For this review, take the finished solid that the model builds, in its own axes (mm). A direction names the side the tool comes from. Coordinates: 2 decimals unless noted, no trailing zeros. Order: outer loops, then holes, each group sorted by start corner. A loop starts at its lowest first (then second) coordinate and runs counter-clockwise, first axis right, second up. Notation, with made-up numbers: (78, 26) - (133, 26) arc R37 cw to (133, 62) - close; hole circle Ø6 at (40, 33). An arc over 180 degrees is marked (long way). One line per item, written item: value. Start each with the question number.
(1) Consider section B-B on z = 50.5. Write out the cut boundary in (x, y), then the cut area to 3 significant figures.
(2) To check wall thickness, follow line 1 along X through (y, z) = (9.5, 38); line 2 along Z through (x, y) = (-91.5, 3.5); line 3 along X through (y, z) = (30.5, 66.5). State the ranges of each line that lie inside material, in increasing order.
(3) For faces 4 (the flat face through (-119, 37, 75)), 5 (the flat face through (-120, 31, 16.891)), 6 (the flat face through (-95, 23.75, 66)), 7 (the flat face through (-92.412, 11.4, 31.9)), 8 (the flat face through (-138.162, 20, 46)), list the 3-axis set-ups (+Z, -Z, +X, -X, +Y, -Y) from which the entire face can be reached by the end or side of a thin tool; tool diameter is ignored.
(4) Consider section D-D on z = 19.5. Count the separate pieces of the cut face and the enclosed holes in it, then the cut area to 3 significant figures.
(5) Mouldability with a two-part tool opening along X and no side actions: class faces 1 (the flat face through (-136.412, 5, 10)), 2 (the flat face through (-113, 11, 74.391)), 3 (the flat face through (-93, 32, 16.641)) as released by +X, released by -X, zero draft, split by the parting line, or undercut.
(6) Consider section C-C on x = -152. Write out the cut boundary in (y, z), then the cut area to 3 significant figures.
(7) Consider section A-A on y = 34. Write out the cut boundary in (x, z), then the cut area to 3 significant figures.
(8) Clearance check with flat-ended pins moving along their axes: pin 1 (12 mm diameter, centred on y = 33, z = 60.5, fed in from +X); pin 2 (12 mm diameter, centred on x = -127, y = 30, fed in from +Z); pin 3 (8 mm diameter, centred on x = -114.5, y = 32.5, fed in from -Z); pin 4 (3 mm diameter, centred on x = -140.5, y = 32, fed in from -Z). State where each tip first meets the part, or that it passes through.
```python
from build123d import *

# Parameters (mm, degrees)
SKETCH1_W               = 49.5
SKETCH1_H               = 61.5
BOSS_EXTRUDE1_DEPTH     = 23.75
SKETCH2_W               = 46
SKETCH2_H               = 58
CUT_EXTRUDE1_DEPTH      = 22
SKETCH3_W               = 3
SKETCH3_H               = 16
CUT_EXTRUDE2_DEPTH      = 1.75
SKETCH7_W               = 3
SKETCH7_H               = 5
BOSS_EXTRUDE2_DEPTH     = 6
SKETCH11_W              = 37.5
SKETCH11_H              = 61.5
BOSS_EXTRUDE3_DEPTH     = 15
SKETCH12_W              = 34.5
SKETCH12_H              = 57
CUT_EXTRUDE3_DEPTH      = 15
SKETCH14_W              = 7.75
SKETCH14_H              = 9
BOSS_EXTRUDE4_DEPTH     = 0.0001
SKETCH15_W              = 4.15
SKETCH15_H              = 5.2
CUT_EXTRUDE4_DEPTH      = 4.75
SKETCH16_W              = 8.5
SKETCH16_H              = 15.5
BOSS_EXTRUDE5_DEPTH     = 16.75
SKETCH17_W              = 5.125
SKETCH17_H              = 6.625
CUT_EXTRUDE5_DEPTH      = 8.5
CUT_EXTRUDE6_DEPTH      = 15
CUT_EXTRUDE6_DEPTH_BACK = 1.75
SKETCH18_W              = 5
SKETCH18_H              = 12
SKETCH20_W              = 16
SKETCH20_H              = 3
CUT_EXTRUDE7_DEPTH      = 1.75
SKETCH21_W              = 32.25
SKETCH21_H              = 81.5
BOSS_EXTRUDE7_DEPTH     = 10
SKETCH23_W              = 28.75
SKETCH23_H              = 78
CUT_EXTRUDE8_DEPTH      = 10
SKETCH25_W              = 3
SKETCH25_H              = 5.4
BOSS_EXTRUDE8_DEPTH     = 1.75
SKETCH28_W              = 3
SKETCH28_H              = 2
BOSS_EXTRUDE9_DEPTH     = 1.75
SKETCH30_W              = 5
SKETCH30_H              = 1.5
BOSS_EXTRUDE11_DEPTH    = 1
SKETCH32_W              = 10.5
SKETCH32_H              = 2.25
CUT_EXTRUDE9_DEPTH      = 1.75
SKETCH33_W              = 11
SKETCH33_H              = 11
CUT_EXTRUDE10_DEPTH     = 1
SKETCH34_W              = 11
SKETCH34_H              = 1
BOSS_EXTRUDE12_DEPTH    = 2


with BuildPart() as part:
    # Sketch1 → Boss-Extrude1 (new body)
    with BuildSketch(Plane(origin=(0, 0, 0), x_dir=(1, 0, 0), z_dir=(0, 1, 0))):
        with Locations((-113.412024913, -45.391200727)):
            Rectangle(SKETCH1_W, SKETCH1_H)
    extrude(amount=BOSS_EXTRUDE1_DEPTH)

    # Sketch2 → Cut-Extrude1 (cut)
    with BuildSketch(Plane(origin=(0, 0, 0), x_dir=(-1, 0, 0), z_dir=(0, -1, 0))):
        with Locations((113.412024913, -45.391200727)):
            Rectangle(SKETCH2_W, SKETCH2_H)
    extrude(amount=-CUT_EXTRUDE1_DEPTH, mode=Mode.SUBTRACT)

    # Sketch3 → Cut-Extrude2 (cut)
    with BuildSketch(Plane(origin=(0, 22, 0), x_dir=(-1, 0, 0), z_dir=(0, -1, 0))):
        with Locations((91.912024913, -66.391200727)):
            Rectangle(SKETCH3_W, SKETCH3_H)
        with Locations((91.912024913, -24.391200727)):
            Rectangle(SKETCH3_W, SKETCH3_H)
        with Locations((91.912024913, -45.391200727)):
            Rectangle(SKETCH3_W, SKETCH3_H)
    extrude(amount=-CUT_EXTRUDE2_DEPTH, mode=Mode.SUBTRACT)

    # Sketch7 → Boss-Extrude2 (add)
    with BuildSketch(Plane(origin=(0, 22, 0), x_dir=(-1, 0, 0), z_dir=(0, -1, 0))):
        with Locations((91.912024913, -55.891200727)):
            Rectangle(SKETCH7_W, SKETCH7_H)
        with Locations((91.912024913, -34.891200727)):
            Rectangle(SKETCH7_W, SKETCH7_H)
    extrude(amount=BOSS_EXTRUDE2_DEPTH)

    # Sketch11 → Boss-Extrude3 (add)
    with BuildSketch(Plane(origin=(0, 23.75, 0), x_dir=(1, 0, 0), z_dir=(0, 1, 0))):
        with Locations((-119.412024913, -45.391200727)):
            Rectangle(SKETCH11_W, SKETCH11_H)
    extrude(amount=BOSS_EXTRUDE3_DEPTH)

    # Sketch12 → Cut-Extrude3 (cut)
    with BuildSketch(Plane(origin=(0, 38.75, 0), x_dir=(1, 0, 0), z_dir=(0, 1, 0))):
        with Locations((-119.412024913, -45.391200727)):
            Rectangle(SKETCH12_W, SKETCH12_H)
    extrude(amount=-CUT_EXTRUDE3_DEPTH, mode=Mode.SUBTRACT)

    # Sketch14 → Boss-Extrude4 (add)
    with BuildSketch(Plane(origin=(0, 23.75, 0), x_dir=(1, 0, 0), z_dir=(0, 1, 0))):
        with Locations((-92.542024913, -66.391200727)):
            Rectangle(SKETCH14_W, SKETCH14_H)
    extrude(amount=BOSS_EXTRUDE4_DEPTH)

    # Sketch15 → Cut-Extrude4 (cut)
    with BuildSketch(Plane(origin=(0, 23.7501, 0), x_dir=(1, 0, 0), z_dir=(0, 1, 0))):
        with Locations((-92.542024913, -66.391200727)):
            Rectangle(SKETCH15_W, SKETCH15_H)
    extrude(amount=-CUT_EXTRUDE4_DEPTH, mode=Mode.SUBTRACT)

    # Sketch16 → Boss-Extrude5 (add)
    with BuildSketch(Plane(origin=(0, 23.75, 0), x_dir=(1, 0, 0), z_dir=(0, 1, 0))):
        with Locations((-92.912024913, -24.391200727)):
            Rectangle(SKETCH16_W, SKETCH16_H)
    extrude(amount=BOSS_EXTRUDE5_DEPTH)

    # Sketch17 → Cut-Extrude5 (cut)
    with BuildSketch(Plane(origin=(-88.662024913, 0, 0), x_dir=(0, 0, -1), z_dir=(1, 0, 0))):
        with Locations((-27.828700727, 35.4375)):
            Rectangle(SKETCH17_W, SKETCH17_H)
        with Locations((-27.828700727, 27.0625)):
            Rectangle(SKETCH17_W, SKETCH17_H)
        with Locations((-20.953700727, 35.4375)):
            Rectangle(SKETCH17_W, SKETCH17_H)
        with Locations((-20.953700727, 27.0625)):
            Rectangle(SKETCH17_W, SKETCH17_H)
    extrude(amount=-CUT_EXTRUDE5_DEPTH, mode=Mode.SUBTRACT)

    # Sketch18 → Cut-Extrude6 (cut, two sides: drawn at the far end of the back side and taken through both)
    with BuildSketch(Plane(origin=(0, 23.75, 0), x_dir=(1, 0, 0), z_dir=(0, 1, 0)).offset(-CUT_EXTRUDE6_DEPTH_BACK)):
        with Locations((-92.912024913, -24.391200727)):
            Rectangle(SKETCH18_W, SKETCH18_H)
    extrude(amount=CUT_EXTRUDE6_DEPTH + CUT_EXTRUDE6_DEPTH_BACK, mode=Mode.SUBTRACT)

    # Sketch20 → Cut-Extrude7 (cut)
    with BuildSketch(Plane(origin=(-100.662024913, 0, 0), x_dir=(0, 0, -1), z_dir=(1, 0, 0))):
        with Locations((-45.391200727, 25.25)):
            Rectangle(SKETCH20_W, SKETCH20_H)
    extrude(amount=-CUT_EXTRUDE7_DEPTH, mode=Mode.SUBTRACT)

    # Sketch21 → Boss-Extrude7 (add)
    with BuildSketch(Plane(origin=(0, 0, 0), x_dir=(-1, 0, 0), z_dir=(0, -1, 0))):
        with Locations((152.537024913, -45.391200727)):
            Rectangle(SKETCH21_W, SKETCH21_H)
    extrude(amount=-BOSS_EXTRUDE7_DEPTH)

    # Sketch23 → Cut-Extrude8 (cut)
    with BuildSketch(Plane(origin=(0, 10, 0), x_dir=(1, 0, 0), z_dir=(0, 1, 0))):
        with Locations((-152.537024913, -45.391200727)):
            Rectangle(SKETCH23_W, SKETCH23_H)
    extrude(amount=-CUT_EXTRUDE8_DEPTH, mode=Mode.SUBTRACT)

    # Sketch25 → Boss-Extrude8 (add)
    with BuildSketch(Plane(origin=(0, 22, 0), x_dir=(-1, 0, 0), z_dir=(0, -1, 0))):
        with Locations((91.912024913, -61.091200727)):
            Rectangle(SKETCH25_W, SKETCH25_H)
        with Locations((91.912024913, -71.691200727)):
            Rectangle(SKETCH25_W, SKETCH25_H)
    extrude(amount=-BOSS_EXTRUDE8_DEPTH)

    # Sketch28 → Boss-Extrude9 (add)
    with BuildSketch(Plane(origin=(0, 23.75, 0), x_dir=(1, 0, 0), z_dir=(0, 1, 0))):
        with Locations((-91.912024913, -17.391200727)):
            Rectangle(SKETCH28_W, SKETCH28_H)
        with Locations((-91.912024913, -31.391200727)):
            Rectangle(SKETCH28_W, SKETCH28_H)
    extrude(amount=-BOSS_EXTRUDE9_DEPTH)

    # Sketch30 → Boss-Extrude11 (add)
    with BuildSketch(Plane.ZY.offset(93.412024913)):
        with Locations((55.891200727, 16.75)):
            Rectangle(SKETCH30_W, SKETCH30_H)
        with Locations((34.891200727, 16.75)):
            Rectangle(SKETCH30_W, SKETCH30_H)
    extrude(amount=BOSS_EXTRUDE11_DEPTH)

    # Sketch32 → Cut-Extrude9 (cut)
    with BuildSketch(Plane(origin=(0, 38.75, 0), x_dir=(1, 0, 0), z_dir=(0, 1, 0))):
        with Locations((-119.412024913, -75.016200727)):
            Rectangle(SKETCH32_W, SKETCH32_H)
        with Locations((-119.412024913, -15.766200727)):
            Rectangle(SKETCH32_W, SKETCH32_H)
    extrude(amount=-CUT_EXTRUDE9_DEPTH, mode=Mode.SUBTRACT)

    # Sketch33 → Cut-Extrude10 (cut)
    with BuildSketch(Plane.ZY.offset(90.412024913)):
        with Locations((32.891200727, 5.5)):
            Rectangle(SKETCH33_W, SKETCH33_H)
    extrude(amount=-CUT_EXTRUDE10_DEPTH, mode=Mode.SUBTRACT)

    # Sketch34 → Boss-Extrude12 (add)
    with BuildSketch(Plane.ZY.offset(90.412024913)):
        with Locations((32.891200727, 11.5)):
            Rectangle(SKETCH34_W, SKETCH34_H)
        Polygon((38.391200727, 12), (38.391200727, 11), (38.391200727, 0), (39.391200727, 0), (39.391200727, 12), align=None)
        Polygon((26.391200727, 0), (27.391200727, 0), (27.391200727, 11), (27.391200727, 12), (26.391200727, 12), align=None)
    extrude(amount=BOSS_EXTRUDE12_DEPTH)


solid = part.part
```
Geometry check:
1. outline: (-168.66, 0) - (-166.91, 0) - (-166.91, 10) - (-168.66, 10) - close; (-138.16, 0) - (-136.41, 0) - (-136.41, 22) - (-93.41, 22) - (-93.41, 23.75) - (-136.66, 23.75) - (-136.66, 38.75) - (-138.16, 38.75) - close; (-102.16, 26.75) - (-100.66, 26.75) - (-100.66, 38.75) - (-102.16, 38.75) - close; (-90.41, 0) - (-88.66, 0) - (-88.66, 23.75) - (-90.41, 23.75) - close
1. area: 216 mm^2
2. line 1: x = -168.66 to -166.91, -138.16 to -136.41, -89.41 to -88.66
2. line 2: z = 14.64 to 16.39, 26.39 to 27.39, 38.39 to 39.39, 74.39 to 76.14
2. line 3: x = -138.16 to -136.66, -102.16 to -100.66
3. face 4: +Z, -Z, +Y
3. face 5: +Y
3. face 6: +Z, +X, +Y
3. face 7: -Y
3. face 8: +Y, -Y
4. separate pieces: 6
4. enclosed holes: 0
4. area: 238 mm^2
5. face 1: released by +X
5. face 2: undercut
5. face 3: zero draft
6. outline: (0, 4.64) - (10, 4.64) - (10, 6.39) - (0, 6.39) - close; (0, 84.39) - (10, 84.39) - (10, 86.14) - (0, 86.14) - close
6. area: 35.0 mm^2
7. outline: (-138.16, 14.64) - (-100.66, 14.64) - (-100.66, 76.14) - (-138.16, 76.14) - close; (-97.16, 16.64) - (-88.66, 16.64) - (-88.66, 18.39) - (-97.16, 18.39) - close; (-97.16, 23.52) - (-95.41, 23.52) - (-95.41, 25.27) - (-97.16, 25.27) - close; (-97.16, 30.39) - (-88.66, 30.39) - (-88.66, 32.14) - (-97.16, 32.14) - close; (-90.41, 23.52) - (-88.66, 23.52) - (-88.66, 25.27) - (-90.41, 25.27) - close; hole (-136.66, 16.89) - (-102.16, 16.89) - (-102.16, 73.89) - (-136.66, 73.89) - close
7. area: 376 mm^2
8. pin 1: stops at x = -100.66
8. pin 2: stops at z = 76.14
8. pin 3: stops at z = 14.64
8. pin 4: passes through
